The listing builds one solid part. Answer for the finished solid, in the listing's coordinates (mm). Round coordinates to 2 decimals unless told otherwise and drop trailing zeros. Loops run counter-clockwise (first coordinate to the right, second up) from the corner with the lowest first, then second, coordinate; pieces in that order, holes last. Notation, with made-up numbers: (-8.5, -25) - (35.5, -25) arc R27 cw to (35.5, -7) - close; hole circle Ø9 at (-9.75, 86.25). An arc over 180 degrees is marked (long way). One line per item, written item: value.
```python
from build123d import *

# Parameters (mm, degrees)
F0_R     = 3.25
F1_DEPTH = 3


# Not quite as in the source:
# - a feature names something its author has since deleted; it is built from what else it names


with BuildPart() as f1:
    # F0 (on Top) → F1 (new body)
    with BuildSketch(Plane.XY):
        Polygon((0, 7), (0, 0), (17, 0), (17, -3), (27, -3), (27, 0), (36, 0), (36, 6.5), (35, 6.5), (35, 8.5), (36, 8.5), (36, 15), (38, 15), (38, 8.5), (39, 8.5), (39, 6.5), (38, 6.5), (38, 0), (47, 0), (47, -3), (57, -3), (57, 0), (66, 0), (66, 6.5), (65, 6.5), (65, 8.5), (66, 8.5), (66, 15), (68, 15), (68, 8.5), (69, 8.5), (69, 6.5), (68, 6.5), (68, 0), (77, 0), (77, -3), (87, -3), (87, 0), (104, 0), (104, 7), (107, 7), (107, 17), (104, 17), (104, 24), (107, 24), (107, 34), (104, 34), (104, 41), (87, 41), (87, 44), (77, 44), (77, 41), (68, 41), (68, 34.5), (69, 34.5), (69, 32.5), (68, 32.5), (68, 26), (66, 26), (66, 32.5), (65, 32.5), (65, 34.5), (66, 34.5), (66, 41), (57, 41), (57, 44), (47, 44), (47, 41), (38, 41), (38, 34.5), (39, 34.5), (39, 32.5), (38, 32.5), (38, 26), (36, 26), (36, 32.5), (35, 32.5), (35, 34.5), (36, 34.5), (36, 41), (27, 41), (27, 44), (17, 44), (17, 41), (0, 41), (0, 34), (-3, 34), (-3, 24), (0, 24), (0, 17), (-3, 17), (-3, 7), align=None)
        with Locations((85.7752785087, 20.5)):
            Circle(F0_R, mode=Mode.SUBTRACT)
    extrude(amount=F1_DEPTH)


solid = f1.part
```
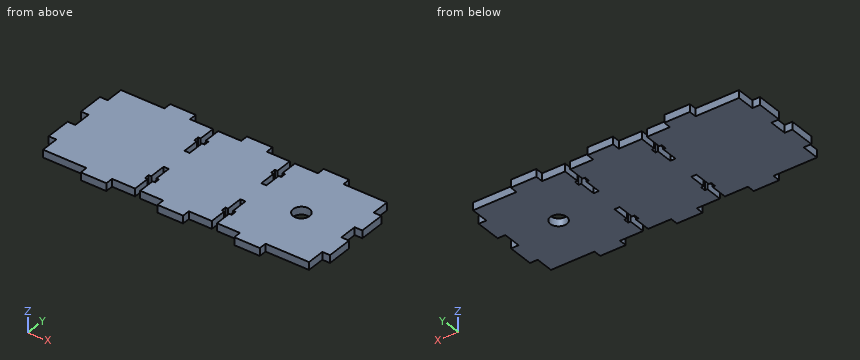
1) A cutting plane is placed at B-B on y = 1. Give the vertices of the cut face in (x, z).
Final values:
outline: (0, 0) - (36, 0) - (36, 3) - (0, 3) - close; (38, 0) - (66, 0) - (66, 3) - (38, 3) - close; (68, 0) - (104, 0) - (104, 3) - (68, 3) - close
2) Each of these flat-tipped pins is pushed along its axis until it touches: pin 1 Ø0.9 at (y, z) = (39, 1.5) entering from -X; pin 2 Ø0.9 at (y, z) = (-2, 1.5) entering from -X; pin 3 Ø1.1 at (x, z) = (38.5, 2) entering from -Y. Where does it stop, or does it pass through?
Final values:
pin 1: x = 0
pin 2: x = 17
pin 3: y = 0
3) A cutting plane is placed at C-C on y = 28. Give the vertices of the cut face in (x, z).
Final values:
outline: (-3, 0) - (36, 0) - (36, 3) - (-3, 3) - close; (38, 0) - (66, 0) - (66, 3) - (38, 3) - close; (68, 0) - (107, 0) - (107, 3) - (68, 3) - close
4) A cutting plane is placed at A-A on y = 20.5. Give the vertices of the cut face in (x, z).
Final values:
outline: (0, 0) - (82.53, 0) - (82.53, 3) - (0, 3) - close; (89.03, 0) - (104, 0) - (104, 3) - (89.03, 3) - close
5) Consider L1, parallel to X at y = 8, z = 2.7; L2, parallel to X at y = 9, z = 2.95; L3, parallel to Y at x = 35.5, z = 2.55. Determine where each line is inside the solid, lowest interval first.
Final values:
L1: -3 to 35, 39 to 65, 69 to 107
L2: -3 to 36, 38 to 66, 68 to 107
L3: 0 to 6.5, 8.5 to 32.5, 34.5 to 41
6) A cutting plane is placed at D-D on x = 30. Give the vertices of the cut face in (y, z), and give its area (3 significant figures).
Final values:
outline: (0, 0) - (41, 0) - (41, 3) - (0, 3) - close
area: 123 mm2
